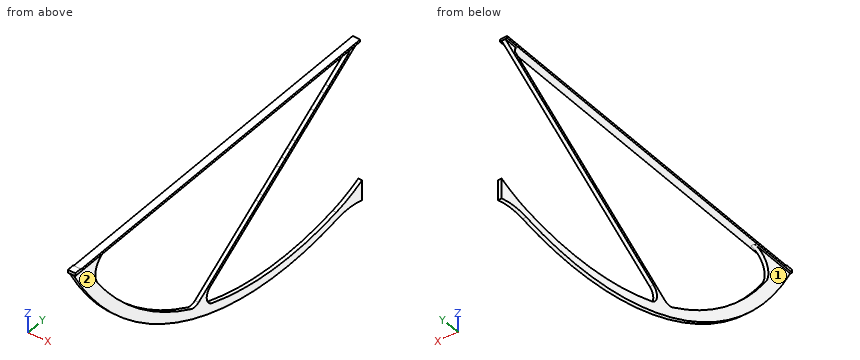
```python
from build123d import *

# Parameters (mm, degrees)
F0_W        = 10
F0_H        = 3
F1_DEPTH    = 505
F3_DEPTH    = 2.5
F4_W        = 10
F4_H        = 9.3853771687
F5_DEPTH    = 1
F6_R        = 13.8620559507
F7_T1_DEPTH = 5
F8_T1_DEPTH = 5
F9_T1_DEPTH = 5
F10_R       = 3.9335934118


# Not quite as in the source:
# - a fillet or chamfer that OpenCascade refuses, or shapes differently, is made with other operations: its cross-section is extruded or revolved along the edge and cut away or added


with BuildPart() as f1:
    # F0 (on Front) → F1 (new body)
    with BuildSketch(Plane.XZ):
        with Locations((0, -9.24)):
            Rectangle(F0_W, F0_H)
    extrude(amount=F1_DEPTH)

    # F2 (on Right) → F3 (join, symmetric)
    with BuildSketch(Plane.YZ):
        with BuildLine():
            Line((-485, -10.74), (-505, -10.74))
            ThreePointArc((-505, -10.74), (-493.7857076195, -12.9341617837), (-482.5908295993, -15.2253199277))
            ThreePointArc((-482.5908295993, -15.2253199277), (-483.8023342329, -12.9863765535), (-485, -10.74))
        make_face()
        with BuildLine():
            ThreePointArc((-482.5908295993, -15.2253199277), (-493.7857076195, -12.9341617837), (-505, -10.74))
            ThreePointArc((-505, -10.74), (-295.8735946629, -205.4541731306), (-10.8822178841, -226.1272906733))
            Line((-10.8822178841, -226.1272906733), (-10.8822178841, -215.5293727716))
            ThreePointArc((-10.8822178841, -215.5293727716), (-149.5821295238, -229.2858372659), (-284.9469559253, -196.0703351995))
            ThreePointArc((-284.9469559253, -196.0703351995), (-287.1338212994, -195.111371401), (-289.3150994302, -194.1397657983))
            ThreePointArc((-289.3150994302, -194.1397657983), (-400.6140653387, -120.5204756417), (-482.5908295993, -15.2253199277))
        make_face()
        with BuildLine():
            Line((-175.5948523726, -120.1757838434), (-289.3150994302, -194.1397657983))
            ThreePointArc((-289.3150994302, -194.1397657983), (-287.1338212994, -195.111371401), (-284.9469559253, -196.0703351995))
            Line((-284.9469559253, -196.0703351995), (-164.6339868931, -117.8184275517))
            Line((-164.6339868931, -117.8184275517), (0, -10.74))
            Line((0, -10.74), (-7.3364102674, -10.74))
            Line((-7.3364102674, -10.74), (-52.0490416838, -39.8212265081))
            Line((-52.0490416838, -39.8212265081), (-59.8008067738, -44.8629972399))
            Line((-59.8008067738, -44.8629972399), (-69.1519232492, -50.9449907999))
            Line((-69.1519232492, -50.9449907999), (-78.2792164974, -56.881409077))
            Line((-78.2792164974, -56.881409077), (-110.8941655597, -78.0942675285))
            Line((-110.8941655597, -78.0942675285), (-120.0217871415, -84.0308993547))
            Line((-120.0217871415, -84.0308993547), (-129.6997254261, -90.3254587772))
            Line((-129.6997254261, -90.3254587772), (-138.8888255597, -96.3020764336))
            Line((-138.8888255597, -96.3020764336), (-168.8523264487, -115.7904252229))
            Line((-168.8523264487, -115.7904252229), (-175.5948523726, -120.1757838434))
        make_face()
        Polygon((-10.8822178841, -215.5293727716), (-10.8822178841, -226.1272906733), (6.6898409277, -234.5661967993), (6.6898409277, -207.0904666456), align=None)
    extrude(amount=F3_DEPTH, both=True)

    # F4 (on face) → F5 (join)
    with BuildSketch(Plane.XY.offset(-7.74)):
        with Locations((0, -500.3073114157)):
            Rectangle(F4_W, F4_H)
    extrude(amount=F5_DEPTH)

    # F6
    f6_edges = [f1.edges().sort_by_distance(p)[0] for p in [
        (0, -284.946956, -196.070335),
        (0, -289.315099, -194.139766),
    ]]
    fillet(f6_edges, radius=F6_R)

    # F7: fillet of radius 24.5086487231 on 1 edges, made by hand

    # F7_s2 → F7_t1 (join)
    with BuildSketch(Plane.YZ.offset(-2.5)):
        with BuildLine():
            ThreePointArc((-441.73429524, -10.74), (-463.3828258275, -23.7588712825), (-462.0321746683, -48.9843668676))
            ThreePointArc((-462.0321746683, -48.9843668676), (-474.0334147231, -30.1728667078), (-485, -10.74))
            Line((-485, -10.74), (-441.73429524, -10.74))
        make_face()
    extrude(amount=F7_T1_DEPTH)

    # F8: fillet of radius 198.8084962623 on 1 edges, made by hand

    # F8_s2 → F8_t1 (join)
    with BuildSketch(Plane.YZ.offset(-2.5)):
        with BuildLine():
            ThreePointArc((-38.9541818345, -222.2094923529), (-15.6734102854, -216.0349668625), (6.6898409277, -207.0904666456))
            Line((6.6898409277, -207.0904666456), (-10.8822178841, -215.5293727716))
            ThreePointArc((-10.8822178841, -215.5293727716), (-24.8597763304, -219.11494661), (-38.9541818345, -222.2094923529))
        make_face()
    extrude(amount=F8_T1_DEPTH)

    # F9: fillet of radius 87.6851690928 on 1 edges, made by hand

    # F9_s2 → F9_t1 (join)
    with BuildSketch(Plane.YZ.offset(-2.5)):
        with BuildLine():
            ThreePointArc((6.6898409277, -234.5661967993), (-15.0768754349, -230.7023497098), (-37.1181822791, -232.4053024821))
            ThreePointArc((-37.1181822791, -232.4053024821), (-23.9509608314, -229.4720686048), (-10.8822178841, -226.1272906733))
            Line((-10.8822178841, -226.1272906733), (6.6898409277, -234.5661967993))
        make_face()
    extrude(amount=F9_T1_DEPTH)

    # F10
    f10_edges = [f1.edges().sort_by_distance(p)[0] for p in [
        (0, -7.33641, -10.74),
    ]]
    fillet(f10_edges, radius=F10_R)


solid = f1.part
```
Check sheet for the modelled part. Datum: model origin and axes. Units: mm. Face numbers are marked on the shaded views. A direction names the side the tool comes from. Round coordinates to 2 decimals unless told otherwise and drop trailing zeros. Order: outer loops, then holes, each group sorted by start corner. A loop starts at its lowest first (then second) coordinate and runs counter-clockwise, first axis right, second up. Notation, with made-up numbers: (48, 42) -> (80, 42) arc R17 cw to (80, 46) -> close; hole circle Ø11 at (83, -34). An arc over 180 degrees is marked (long way). One line per item, written item: value. Start each with the question number.
Q1. Thickness scan on line 1 (Z direction, x = 0.75, y = -90); line 2 (Z direction, x = 3.5, y = -383); line 3 (Z direction, x = 1, y = -378). Record the ranges inside material, lowest first.
Q2. Cross-section at A-A (y = -274.5). Record the boundary of the cut face in (x, z).
Q3. Gauge pin test, flat ends, axial feed: pin 1 Ø6 at (x, y) = (1.5, -93.5) entering from -Z; pin 2 Ø0.8 at (x, z) = (-0.5, -7.5) entering from +Y; pin 3 Ø1.5 at (y, z) = (-349, -172.5) entering from -X. Record the tip position at first contact, or that the pin passes through.
Q4. Cross-section at D-D (z = -200.5). Record the boundary of the cut face in (x, y), and give its area (3 significant figures).
Q5. Cross-section at B-B (z = -26). Record the boundary of the cut face in (x, y), and give its area (3 significant figures).
Q6. Cross-section at C-C (x = 0). Record the boundary of the cut face in (y, z), and give its area (3 significant figures).
Q7. Set-up check for the marked faces 1 and 2: record each of +Z, -Z, +X, -X, +Y, -Y from which the full face is reachable in a straight line by a thin tool's end or side.
Completed:
1. line 1: z = -239.93 to -229.2, -69.28 to -64.5, -10.74 to -7.74
1. line 2: z = -10.74 to -7.74
1. line 3: z = -158.28 to -139.98, -10.74 to -7.74
2. outline: (-5, -10.74) -> (5, -10.74) -> (5, -7.74) -> (-5, -7.74) -> close; (-2.5, -214.1) -> (2.5, -214.1) -> (2.5, -184.5) -> (-2.5, -184.5) -> close
3. pin 1: stops at z = -240.4
3. pin 2: stops at y = 0
3. pin 3: stops at x = -2.5
4. outline: (-2.5, -306.82) -> (2.5, -306.82) -> (2.5, -266.61) -> (-2.5, -266.61) -> close
4. area: 201 mm²
5. outline: (-2.5, -496.61) -> (2.5, -496.61) -> (2.5, -464.43) -> (-2.5, -464.43) -> close; (-2.5, -30.8) -> (2.5, -30.8) -> (2.5, -23.46) -> (-2.5, -23.46) -> close
5. area: 198 mm²
6. outline: (-505, -10.74) arc R430.05 ccw to (-37.12, -232.41) arc R87.69 cw to (6.69, -234.57) -> (6.69, -207.09) arc R198.81 cw to (-38.95, -222.21) arc R412.55 cw to (-259.59, -206.12) arc R13.86 cw to (-262.47, -181.45) -> (0, -10.74) -> (0, -7.74) -> (-495.61, -7.74) -> (-495.61, -6.74) -> (-505, -6.74) -> close; hole (-462.03, -48.98) arc R412.55 ccw to (-296.38, -190.89) arc R13.86 ccw to (-282.91, -189.97) -> (-18.45, -17.97) arc R3.93 ccw to (-20.6, -10.74) -> (-441.73, -10.74) arc R24.51 ccw to start
6. area: 11,500 mm²
7. face 1: -Z, -X, +Y, -Y
7. face 2: -Z, +X, +Y, -Y
